Can you work these out from the model? Positions are in its coordinate system, mm. A direction names the side the tool comes from. Give positions to 0.01 mm unless a question says otherwise; leave off trailing zeros. Write each loop counter-clockwise with the first axis right and the second up, starting at its lowest first coordinate (ties: lowest second). Pieces come first, ordered by that corner, then holes.
from build123d import *

# Parameters (mm, degrees)
ESQUISSE1_W             = 6
ESQUISSE1_H             = 9.5
ESQUISSE2_W             = 3
ESQUISSE2_H             = 6
ENL_V_MAT_EXTRU_1_DEPTH = 10
ESQUISSE3_W             = 3
ESQUISSE3_H             = 6
ENL_V_MAT_EXTRU_2_DEPTH = 10


with BuildPart() as part:
    # Esquisse1 → Base-Révolution (revolve)
    with BuildSketch(Plane.XY, mode=Mode.PRIVATE) as base_r_volution_sk:
        with Locations((3, 4.75)):
            Rectangle(ESQUISSE1_W, ESQUISSE1_H)
    revolve(base_r_volution_sk.sketch.rotate(Axis((0, 0, 0), (1, 0, 0)), 90), axis=Axis((0, 0, 0), (1, 0, 0)))

    # Esquisse2 → Enlèv. mat.-Extru.1 (cut, symmetric)
    with BuildSketch(Plane.XY):
        with Locations((1.5, 0)):
            Rectangle(ESQUISSE2_W, ESQUISSE2_H)
    extrude(amount=ENL_V_MAT_EXTRU_1_DEPTH, both=True, mode=Mode.SUBTRACT)

    # Esquisse3 → Enlèv. mat.-Extru.2 (cut, symmetric)
    with BuildSketch(Plane(origin=(0, 0, 0), x_dir=(1, 0, 0), z_dir=(0, 1, 0))):
        with Locations((4.5, 0)):
            Rectangle(ESQUISSE3_W, ESQUISSE3_H)
    extrude(amount=ENL_V_MAT_EXTRU_2_DEPTH, both=True, mode=Mode.SUBTRACT)


solid = part.part
(1) Will these pins go through, and if not, where does the flat tip stop? P1, Ø5, axis at y = 7.5, z = 1.5, coming from the -X side; P2, Ø1.5, axis at x = 5, y = -1.5, coming from the +Z side; P3, Ø0.9, axis at x = 4.5, y = -2, coming from the -Z side; P4, Ø1, axis at y = 1, z = -1.5, coming from the -X side.
Returned:
P1: stops at x = 0
P2: stops at z = 9.47
P3: stops at z = -9.37
P4: passes through
(2) Imagine slicing it at A-A, the plane z = 0. Write out the boundary of the cut face in (x, y).
Returned:
outline: (0, -9.5) - (3, -9.5) - (3, -3) - (0, -3) - close; (0, 3) - (3, 3) - (3, 9.5) - (0, 9.5) - close
(3) If I drill on L1, parallel to X at y = -2.75, z = 8; L2, parallel to Z at x = 5.75, y = -6.25; L3, parallel to Z at x = 3.85, y = 8.5, over which ranges is the centre line in solid material (lowest first)?
Returned:
L1: x = 3 to 6
L2: z = -7.15 to -3, 3 to 7.15
L3: z = -4.24 to -3, 3 to 4.24
(4) Imagine slicing it at D-D, the plane z = 8.5. Write out the boundary of the cut face in (x, y), plus the area to 3 significant figures.
Returned:
outline: (0, -4.24) - (6, -4.24) - (6, 4.24) - (0, 4.24) - (0, 3) - (3, 3) - (3, -3) - (0, -3) - close
area: 32.9 mm2
(5) If we mould it in two halves opening along Z, with no side actions, what happens to faces 4 (the face through (3.042, 3.639, 8.776)), 5 (the face through (0, 5, 0)), 6 (the face through (3, 6, 0))? For each: +Z half, -Z half, draft (parallel to the pull), parting line (faces both ways), or undercut.
Returned:
face 4: parting line
face 5: draft
face 6: undercut
(6) For faces 1 (the face through (4, 0, -3)), 2 (the face through (3, 0, -6)), 3 (the face through (0, -6, 0)), which set-ups out of +Z, -Z, +X, -X, +Y, -Y let a thin tool reach every point of the face, with its end or its side?
Returned:
face 1: +X, +Y, -Y
face 2: +Z, -Z, -X
face 3: +Z, -Z, -X, +Y, -Y
(7) Imagine slicing it at C-C, the plane x = 4.5. Write out the boundary of the cut face in (y, z), plus the area to 3 significant figures.
Returned:
outline: (-9.01, -3) arc R9.5 ccw to (9.01, -3) - close; (-9.01, 3) - (9.01, 3) arc R9.5 ccw to start
area: 171 mm2
(8) Imagine slicing it at B-B, the plane y = 1.25. Write out the boundary of the cut face in (x, z).
Returned:
outline: (3, -9.42) - (6, -9.42) - (6, -3) - (3, -3) - close; (3, 3) - (6, 3) - (6, 9.42) - (3, 9.42) - close
